from build123d import *

# Parameters (mm, degrees)
F0_R      = 3
F1_DEPTH  = 0.5
F2_R      = 2.499
F2_R_2    = 1.999
F3_DEPTH  = 5.9
F4_R      = 2.75
F4_R_2    = 1.999
F5_DEPTH  = 1
F7_DEPTH  = 3
F9_DEPTH  = 7.4
F10_DEPTH = 0.5
F11_DEPTH = 0.5


with BuildPart() as f1:
    # F0 (on Front) → F1 (new body, symmetric)
    with BuildSketch(Plane.XZ):
        Circle(F0_R)
    extrude(amount=F1_DEPTH, both=True)

    # F2 (on face) → F3 (join)
    with BuildSketch(Plane.XZ.offset(0.5)):
        Circle(F2_R)
        Circle(F2_R_2, mode=Mode.SUBTRACT)
    extrude(amount=F3_DEPTH)

    # F4 (on face) → F5 (join)
    with BuildSketch(Plane.XZ.offset(6.4)):
        Circle(F4_R)
        Circle(F4_R_2, mode=Mode.SUBTRACT)
    extrude(amount=F5_DEPTH)

    # F6 (on face) → F7 (cut)
    with BuildSketch(Plane.XZ.offset(7.4)):
        with BuildLine():
            ThreePointArc((2.7386127875, -0.25), (2.75, 0), (2.7386127875, 0.25))
            Line((2.7386127875, 0.25), (1.983305574, 0.25))
            ThreePointArc((1.983305574, 0.25), (1.999, 0), (1.983305574, -0.25))
            Line((1.983305574, -0.25), (2.7386127875, -0.25))
        make_face()
        with BuildLine():
            Line((-2.7386127875, -0.25), (-1.983305574, -0.25))
            ThreePointArc((-1.983305574, -0.25), (-1.999, 0), (-1.983305574, 0.25))
            Line((-1.983305574, 0.25), (-2.7386127875, 0.25))
            ThreePointArc((-2.7386127875, 0.25), (-2.75, 0), (-2.7386127875, -0.25))
        make_face()
    extrude(amount=-F7_DEPTH, mode=Mode.SUBTRACT)

    # F8 (on face) → F9 (join)
    with BuildSketch(Plane(origin=(0, 0.5, 0), x_dir=(-1, 0, 0), z_dir=(0, 1, 0))):
        with BuildLine():
            Line((-0.9, -0.9), (-0.9, -2.3313088598))
            ThreePointArc((-0.9, -2.3313088598), (0, -2.499), (0.9, -2.3313088598))
            Line((0.9, -2.3313088598), (0.9, -0.9))
            Line((0.9, -0.9), (2.3313088598, -0.9))
            ThreePointArc((2.3313088598, -0.9), (2.499, 0), (2.3313088598, 0.9))
            Line((2.3313088598, 0.9), (0.9, 0.9))
            Line((0.9, 0.9), (0.9, 2.3313088598))
            ThreePointArc((0.9, 2.3313088598), (0, 2.499), (-0.9, 2.3313088598))
            Line((-0.9, 2.3313088598), (-0.9, 0.9))
            Line((-0.9, 0.9), (-2.3313088598, 0.9))
            ThreePointArc((-2.3313088598, 0.9), (-2.499, 0), (-2.3313088598, -0.9))
            Line((-2.3313088598, -0.9), (-0.9, -0.9))
        make_face()
    extrude(amount=F9_DEPTH)

    # F10 (add): faces of the model
    f10_faces = [f1.faces().sort_by_distance(p)[0] for p in [
        (2.3609591808, -7.4, 0.3102079729),
        (0, -7.4, -2.6897920271),
    ]]
    extrude(f10_faces, amount=F10_DEPTH)

    # F11 (cut): faces of the model
    f11_faces = [f1.faces().sort_by_distance(p)[0] for p in [
        (2.6125381702, -6.4, 0.3102079729),
        (0, -6.4, -2.6897920271),
    ]]
    extrude(f11_faces, amount=-F11_DEPTH, mode=Mode.SUBTRACT)


solid = f1.part
Geometry check sheet. Reference: the model listing, model coordinates, mm. A direction names the side the tool comes from. Give positions to 0.01 mm unless a question says otherwise; leave off trailing zeros. Write each loop counter-clockwise with the first axis right and the second up, starting at its lowest first coordinate (ties: lowest second). Pieces come first, ordered by that corner, then holes.
1) Cross-section at B-B (x = 1.15). Record the boundary of the cut face in (y, z).
Values follow:
outline: (-7.9, -2.5) - (-6.9, -2.5) - (-6.9, -2.22) - (-0.5, -2.22) - (-0.5, -2.77) - (0.5, -2.77) - (0.5, -0.9) - (7.9, -0.9) - (7.9, 0.9) - (0.5, 0.9) - (0.5, 2.77) - (-0.5, 2.77) - (-0.5, 2.22) - (-6.9, 2.22) - (-6.9, 2.5) - (-7.9, 2.5) - (-7.9, 1.64) - (-0.5, 1.64) - (-0.5, -1.64) - (-7.9, -1.64) - close
2) Set-up check for faces 1 (the face through (0.06, -7.39, 2.75)), 2 (the face through (-2.5, 4.1, 0)), 3 (the face through (-0.9, 4, 2)): record each of +Z, -Z, +X, -X, +Y, -Y from which the full face is reachable in a straight line by a thin tool's end or side.
Values follow:
face 1: +Z, -Y
face 2: -X, +Y
face 3: +Z, -X, +Y
3) Cross-section at D-D (x = 0). Record the boundary of the cut face in (y, z), plus the area to 3 significant figures.
Values follow:
outline: (-7.9, -2.75) - (-6.9, -2.75) - (-6.9, -2.5) - (-0.5, -2.5) - (-0.5, -3) - (0.5, -3) - (0.5, -2.5) - (7.9, -2.5) - (7.9, 2.5) - (0.5, 2.5) - (0.5, 3) - (-0.5, 3) - (-0.5, 2.5) - (-6.9, 2.5) - (-6.9, 2.75) - (-7.9, 2.75) - (-7.9, 2) - (-0.5, 2) - (-0.5, -2) - (-7.9, -2) - close
area: 50.9 mm2
4) Cross-section at C-C (y = 1). Record the boundary of the cut face in (x, z), plus the area to 3 significant figures.
Values follow:
outline: (-2.33, -0.9) - (-0.9, -0.9) - (-0.9, -2.33) arc R2.5 ccw to (0.9, -2.33) - (0.9, -0.9) - (2.33, -0.9) arc R2.5 ccw to (2.33, 0.9) - (0.9, 0.9) - (0.9, 2.33) arc R2.5 ccw to (-0.9, 2.33) - (-0.9, 0.9) - (-2.33, 0.9) arc R2.5 ccw to start
area: 14.4 mm2
5) Thickness scan on line 1 (X direction, y = -2.5, z = 0); line 2 (Y direction, x = 2.35, z = -0.95). Record the ranges inside material, lowest first.
Values follow:
line 1: x = -2.5 to -2, 2 to 2.5
line 2: y = -7.9 to -6.9, -0.5 to 0.5
6) Release check for a two-part mould opening along Y. For faces 4 (the face through (-2, 4, 0.9)), 5 (the face through (2.384, -3.655, 0.751)), 6 (the face through (0, -0.5, 0)) record: released by +Y, released by -Y, zero draft, split by the parting line, or undercut.
Values follow:
face 4: zero draft
face 5: undercut
face 6: released by -Y
7) Go/stop test with flat-tipped pins: pin 1 Ø1 at (x, y) = (-2, -1.5) entering from -Z; pin 2 Ø0.7 at (y, z) = (3, -2) entering from -X; pin 3 Ø1.1 at (y, z) = (6, -1.5) entering from +X; pin 4 Ø0.6 at (x, z) = (2.5, 0) entering from -Y. Record where each tip stops, or that it passes through.
Values follow:
pin 1: stops at z = -2
pin 2: stops at x = -0.9
pin 3: stops at x = 0.9
pin 4: stops at y = -7.9
8) Cross-section at A-A (z = 0). Record the boundary of the cut face in (x, y).
Values follow:
outline: (-3, -0.5) - (-2.5, -0.5) - (-2.5, -4.4) - (-2, -4.4) - (-2, -0.5) - (2, -0.5) - (2, -4.4) - (2.5, -4.4) - (2.5, -0.5) - (3, -0.5) - (3, 0.5) - (2.5, 0.5) - (2.5, 7.9) - (-2.5, 7.9) - (-2.5, 0.5) - (-3, 0.5) - close
